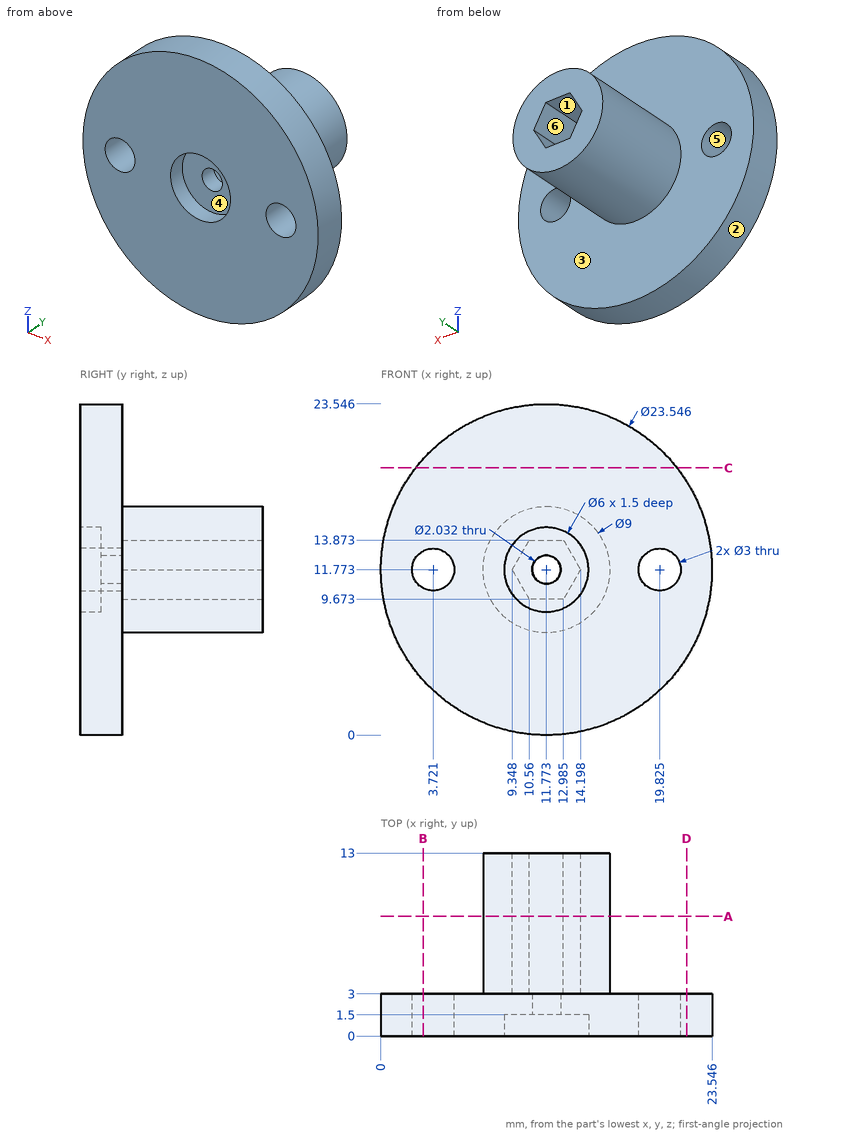
Check sheet for the drawn part. Datum: minimum x, y, z corner. Units: mm. A direction names the side the tool comes from. Coordinates: 2 decimals unless noted, no trailing zeros. Write each loop counter-clockwise with the first axis right and the second up, starting at its lowest first coordinate (ties: lowest second). Pieces come first, ordered by that corner, then holes. Notation, with made-up numbers: (76, -10.75) - (109, -10.75) arc R13 cw to (109, 1.25) - close; hole circle Ø8 at (73.25, 66.25). An arc over 180 degrees is marked (long way). Answer as a JSON object with one key per item and string values.
(1) Gauge pin test, flat ends, axial feed: pin 1 Ø1.5 at (y, z) = (3.5, 21) entering from -X (1 decimal); pin 2 Ø3 at (y, z) = (7, 13) entering from -X; pin 3 Ø6 at (y, z) = (5.5, 14) entering from -X. Record the tip position at first contact, or that the pin passes through.
Report:
{"pin 1": "x = 3.8", "pin 2": "x = 7.27", "pin 3": "x = 0.01"}
(2) Cross-section at C-C on z = 19. Record the cut outline in (x, y).
Report:
{"outline": "(2.48, 0) - (21.07, 0) - (21.07, 3) - (2.48, 3) - close"}
(3) Cross-section at B-B on x = 3. Record the cut outline in (y, z), plus the area to 3 significant figures.
Report:
{"outline": "(0, 3.92) - (3, 3.92) - (3, 10.46) - (0, 10.46) - close; (0, 13.09) - (3, 13.09) - (3, 19.62) - (0, 19.62) - close", "area": "39.2 mm^2"}
(4) Cross-section at D-D on x = 21.75. Record the cut outline in (y, z).
Report:
{"outline": "(0, 5.52) - (3, 5.52) - (3, 18.02) - (0, 18.02) - close"}
(5) Cross-section at A-A on y = 8.5. Record the cut outline in (x, z) (1 decimal).
Report:
{"outline": "circle Ø9 at (11.8, 11.8); hole (9.3, 11.8) - (10.6, 9.7) - (13, 9.7) - (14.2, 11.8) - (13, 13.9) - (10.6, 13.9) - close"}
(6) Mould release check, pull along X, two halves, no side actions. Record for the marked faces 1, 2 and 3: pulls with the +X half, pulls with the -X half, needs draft (parallel to the pull), parting line crosses it, or undercut.
Report:
{"face 1": "undercut", "face 2": "parting line crosses it", "face 3": "needs draft"}
(7) Tool access check on the marked faces 4, 5 and 6. Record the directions out of +Z, -Z, +X, -X, +Y, -Y that give a thin tool (end or side, any length) a straight path to the whole face; none if there is none.
Report:
{"face 4": "-Y", "face 5": "+Y, -Y", "face 6": "+Y"}
(8) Thickness scan on line 1 along Y through (x, z) = (6.5, 5); line 2 along Z through (x, y) = (12.25, 9.25); line 3 along Y through (x, z) = (12.25, 10). Record the ranges inside material, lowest first.
Report:
{"line 1": "0 to 3", "line 2": "7.3 to 9.67, 13.87 to 16.25", "line 3": "1.5 to 3"}
